```python
from build123d import *

# Parameters (mm, degrees)
SKETCH1_W                         = 32
SKETCH1_H                         = 29
BOSS_EXTRUDE1_DEPTH               = 35
FILLET1_R                         = 2
SLOT_FOR_COIL_DEPTH               = 1
SLOT_FOR_COIL_DEPTH_BACK          = 30
BOSS_EXTRUDE2_DEPTH               = 6.5
BOSS_EXTRUDE3_DEPTH               = 1.75
SKETCH5_W                         = 2
SKETCH5_H                         = 6.5
SLOT_TO_FEED_IN_WIRE_DEPTH        = 33
SLOT_FO_PCB_DEPTH                 = 22.5
SKETCH7_W                         = 2
SKETCH7_H                         = 33
BOSS_EXTRUDE4_DEPTH               = 2.5
FILLET2_R                         = 6
ROD_MOUNT_SLOT_REACH              = 34
SKETCH14_W                        = 2.5
SKETCH14_H                        = 20
SIDE_CAVITY_FOR_MOUNT_PLATE_DEPTH = 22.5
SKETCH16_W                        = 2
SKETCH16_H                        = 2
SIDE_STOPS_FOR_MOUNT_PLATE_DEPTH  = 22.5
BOSS_EXTRUDE6_DEPTH               = 22.5
SKETCH21_W                        = 12
SKETCH21_H                        = 2
BOSS_EXTRUDE7_DEPTH               = 4
SKETCH23_W                        = 8
SKETCH23_H                        = 1.75
CUT_EXTRUDE7_DEPTH                = 2
FILLET3_R                         = 1
CUT_EXTRUDE8_REACH                = 34
SKETCH26_R                        = 5.25


with BuildPart() as part:
    # Sketch1 → Boss-Extrude1 (new body)
    with BuildSketch(Plane.XY):
        Rectangle(SKETCH1_W, SKETCH1_H)
    extrude(amount=BOSS_EXTRUDE1_DEPTH)

    # Fillet1
    fillet1_edges = [part.edges().sort_by_distance(p)[0] for p in [
        (16, -14.5, 17.5),
        (-16, -14.5, 17.5),
        (-16, 14.5, 17.5),
        (16, 14.5, 17.5),
    ]]
    fillet(fillet1_edges, radius=FILLET1_R)

    # Sketch2 → Slot for Coil (cut, two sides)
    with BuildSketch(Plane.XZ.offset(14.5)) as slot_for_coil_sk:
        Polygon((-9.125, 0), (-9.125, 1.75), (-11.125, 1.75), (-11.125, 5), (11.125, 5), (11.125, 1.75), (9.125, 1.75), (9.125, 0), align=None)
    extrude(amount=SLOT_FOR_COIL_DEPTH, mode=Mode.SUBTRACT)
    extrude(slot_for_coil_sk.sketch, amount=-SLOT_FOR_COIL_DEPTH_BACK, mode=Mode.SUBTRACT)

    # Sketch3 → Boss-Extrude2 (add)
    with BuildSketch(Plane.XZ.offset(14.5)):
        Polygon((-9.125, 0), (-9.125, 1.75), (-11.125, 1.75), (-11.125, 5), (11.125, 5), (11.125, 1.75), (9.125, 1.75), (9.125, 0), align=None)
    extrude(amount=-BOSS_EXTRUDE2_DEPTH)

    # Sketch4 → Boss-Extrude3 (add)
    with BuildSketch(Plane(origin=(0, 0, 1.75), x_dir=(-1, 0, 0), z_dir=(0, 0, -1))):
        with BuildLine():
            Line((-9.125, 7.5), (-9.125, 6.5))
            ThreePointArc((-9.125, 6.5), (-8.875, 7), (-9.125, 7.5))
        make_face()
    boss_extrude3 = extrude(amount=BOSS_EXTRUDE3_DEPTH)

    # Mirror1: Boss-Extrude3 across plane
    add(boss_extrude3.mirror(Plane(origin=(0, 0, 0), x_dir=(0, 0, 1), z_dir=(1, 0, 0))))

    # Sketch5 → slot to feed in wire (cut)
    with BuildSketch(Plane(origin=(0, 0, 0), x_dir=(-1, 0, 0), z_dir=(0, 0, -1))):
        with Locations((0, -11.25)):
            Rectangle(SKETCH5_W, SKETCH5_H)
    extrude(amount=-SLOT_TO_FEED_IN_WIRE_DEPTH, mode=Mode.SUBTRACT)

    # Sketch6 → slot fo PCB (cut)
    with BuildSketch(Plane(origin=(0, 14.5, 0), x_dir=(1, 0, 0), z_dir=(0, 1, 0))):
        Polygon((11.5, -7.5), (-11.5, -7.5), (-11.5, -29.5), (-12.5, -29.5), (-12.5, -33), (12.5, -33), (12.5, -29.5), (11.5, -29.5), align=None)
    extrude(amount=-SLOT_FO_PCB_DEPTH, mode=Mode.SUBTRACT)

    # Sketch7 → Boss-Extrude4 (add)
    with BuildSketch(Plane.XZ.offset(14.5)):
        with Locations((0, 16.5)):
            Rectangle(SKETCH7_W, SKETCH7_H)
    extrude(amount=-BOSS_EXTRUDE4_DEPTH)

    # Fillet2
    fillet2_edges = [part.edges().sort_by_distance(p)[0] for p in [
        (0, -12, 33),
    ]]
    fillet(fillet2_edges, radius=FILLET2_R)

    # Sketch11 → Rod Mount Slot (cut, up to next)
    with BuildSketch(Plane(origin=(16, 0, 44), x_dir=(0, 0, -1), z_dir=(1, 0, 0)), mode=Mode.PRIVATE) as rod_mount_slot_sk1:
        with BuildLine():
            Line((32.5, 25), (32.5, 0))
            ThreePointArc((32.5, 0), (26.5, -6), (20.5, 0))
            Line((20.5, 0), (20.5, 25))
            ThreePointArc((20.5, 25), (26.5, 31), (32.5, 25))
        make_face()
    rod_mount_slot_tool1 = extrude(rod_mount_slot_sk1.sketch, amount=-ROD_MOUNT_SLOT_REACH, mode=Mode.PRIVATE) & part.part
    add(rod_mount_slot_tool1.solids().sort_by_distance((16, 12.5, 17.5))[0], mode=Mode.SUBTRACT)

    # Sketch14 → Side cavity for mount plate (cut)
    with BuildSketch(Plane(origin=(0, 14.5, 0), x_dir=(1, 0, 0), z_dir=(0, 1, 0))):
        with Locations((12.75, -17.5)):
            Rectangle(SKETCH14_W, SKETCH14_H)
    extrude(amount=-SIDE_CAVITY_FOR_MOUNT_PLATE_DEPTH, mode=Mode.SUBTRACT)

    # Sketch16 → Side stops for mount plate (add)
    with BuildSketch(Plane(origin=(0, 14.5, 0), x_dir=(1, 0, 0), z_dir=(0, 1, 0))):
        with Locations((11, -8.5)):
            Rectangle(SKETCH16_W, SKETCH16_H)
        with Locations((11, -26.5)):
            Rectangle(SKETCH16_W, SKETCH16_H)
    extrude(amount=-SIDE_STOPS_FOR_MOUNT_PLATE_DEPTH)

    # Sketch20 → Boss-Extrude6 (add)
    with BuildSketch(Plane(origin=(0, 14.5, 0), x_dir=(1, 0, 0), z_dir=(0, 1, 0))):
        Polygon((11.5, -29.5), (10, -27.5), (11.5, -27.5), align=None)
        Polygon((10, -9.5), (8.5, -7.5), (10, -7.5), align=None)
    extrude(amount=-BOSS_EXTRUDE6_DEPTH)

    # Sketch21 → Boss-Extrude7 (add)
    with BuildSketch(Plane(origin=(0, 14.5, 0), x_dir=(-1, 0, 0), z_dir=(0, 1, 0))):
        with Locations((0, 34)):
            Rectangle(SKETCH21_W, SKETCH21_H)
    boss_extrude7 = extrude(amount=BOSS_EXTRUDE7_DEPTH)

    # Sketch23 → Cut-Extrude7 (cut)
    with BuildSketch(Plane.XY.offset(35)):
        with Locations((0, 15.875)):
            Rectangle(SKETCH23_W, SKETCH23_H)
    cut_extrude7 = extrude(amount=-CUT_EXTRUDE7_DEPTH, mode=Mode.SUBTRACT)

    # Mirror3: Boss-Extrude7, Cut-Extrude7 across plane
    add(boss_extrude7.mirror(Plane.ZX))
    add(cut_extrude7.mirror(Plane.ZX), mode=Mode.SUBTRACT)

    # Fillet3
    fillet3_edges = [part.edges().sort_by_distance(p)[0] for p in [
        (6, 14.5, 34),
        (-6, 14.5, 34),
        (6, 18.5, 34),
        (-6, 18.5, 34),
        (6, -18.5, 34),
        (-6, -18.5, 34),
        (6, -14.5, 34),
        (-6, -14.5, 34),
    ]]
    fillet(fillet3_edges, radius=FILLET3_R)

    # Sketch26 → Cut-Extrude8 (cut, up to next)
    with BuildSketch(Plane(origin=(-16, 0, 0), x_dir=(0, 0, -1), z_dir=(1, 0, 0)), mode=Mode.PRIVATE) as cut_extrude8_sk1:
        with Locations((-23.015, -2.89)):
            Circle(SKETCH26_R)
    cut_extrude8_tool1 = extrude(cut_extrude8_sk1.sketch, amount=CUT_EXTRUDE8_REACH, mode=Mode.PRIVATE) & part.part
    add(cut_extrude8_tool1.solids().sort_by_distance((-16, -2.89, 23.015))[0], mode=Mode.SUBTRACT)


solid = part.part
```
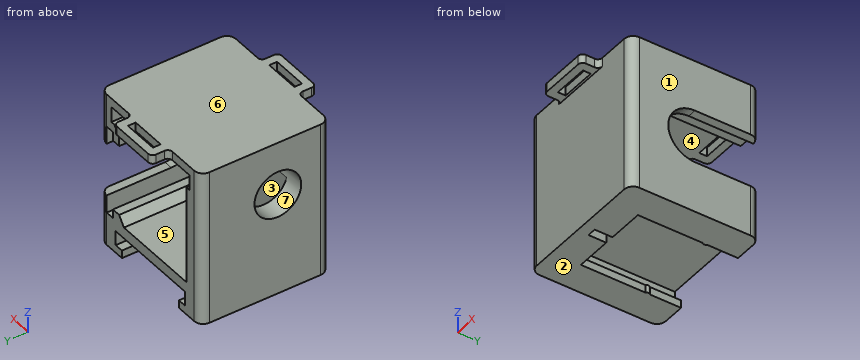
Source: CAD feature listing. Evaluate the final solid. Frame: model axes, mm. Face numbers are marked on the shaded views. A direction names the side the tool comes from. Give positions to 0.01 mm unless a question says otherwise; leave off trailing zeros. Write each loop counter-clockwise with the first axis right and the second up, starting at its lowest first coordinate (ties: lowest second). Pieces come first, ordered by that corner, then holes.
1. Section query A-A (x = -12). Return the cut outline in (y, z) (3 decimals), then the cut area to 3 significant figures.
2. First-contact query: pin 1 (5.5 mm diameter, centred on x = 8.5, z = 2, fed in from +Y); pin 2 (1.5 mm diameter, centred on x = -3, z = 16.5, fed in from +Y); pin 3 (0.5 mm diameter, centred on y = 16, z = 34, fed in from +X). Flat tips, straight axial feed; report the tip coordinate or a pass-through.
3. Section query C-C (x = -2). Return the cut outline in (y, z) (3 decimals), then the cut area to 3 significant figures.
4. Section query D-D (x = 13). Return the cut outline in (y, z).
5. Material intervals for line 1 along Z through (x, y) = (-10.75, -2.89); line 2 along X through (y, z) = (11.5, 8) (3 decimals); line 3 along Z through (x, y) = (-9, -2), sorted ascending.
6. Pull-direction query (Z, two-part tool) for the marked faces 1, 2, 3 and 4; classes: +Z half, -Z half, draft (parallel to the pull), parting line (faces both ways), or undercut.
7. Access query for the marked faces 5, 6 and 7. Directions: +Z, -Z, +X, -X, +Y, -Y. A direction counts if a zero-diameter tool reaches every point of the face in a straight line with its end or side. Return the directions, or none.
Output values:
1. outline: (-14.5, 0) - (14.5, 0) - (14.5, 29.5) - (-8, 29.5) - (-8, 32.657) arc R6 cw to (-6, 33) - (14.5, 33) - (14.5, 35) - (-14.5, 35) - close; hole circle Ø10.5 at (-2.89, 23.015)
1. area: 850 mm2
2. pin 1: stops at y = 14.5
2. pin 2: stops at y = -8
2. pin 3: stops at x = 6
3. outline: (-18.5, 33) - (-16.75, 33) - (-16.75, 35) - (-18.5, 35) - close; (-15, 33) - (-14.5, 33) - (-14.5, 0) - (-8, 0) - (-8, 5) - (14.5, 5) - (14.5, 7.5) - (-8, 7.5) - (-8, 21.811) arc R5.25 cw to (-8, 24.219) - (-8, 32.657) arc R6 cw to (-6, 33) - (15, 33) - (15, 35) - (-15, 35) - close; (16.75, 33) - (18.5, 33) - (18.5, 35) - (16.75, 35) - close
3. area: 338 mm2
4. outline: (-14.5, 0) - (14.5, 0) - (14.5, 7.5) - (-8, 7.5) - (-8, 27.5) - (14.5, 27.5) - (14.5, 35) - (-14.5, 35) - close
5. line 1: z = 0 to 1.75, 5 to 7.5, 33 to 35
5. line 2: x = -16 to -11.5, 8.875 to 12, 14 to 16
5. line 3: z = 5 to 7.5, 33 to 35
6. face 1: draft
6. face 2: -Z half
6. face 3: undercut
6. face 4: undercut
7. face 5: +Y
7. face 6: +Z, +X, -X, +Y, -Y
7. face 7: -X
